Source: CAD feature listing. Evaluate the final solid. Frame: model axes, mm. Face numbers are marked on the shaded views. A direction names the side the tool comes from. Give positions to 0.01 mm unless a question says otherwise; leave off trailing zeros. Order: outer loops, then holes, each group sorted by start corner. A loop starts at its lowest first (then second) coordinate and runs counter-clockwise, first axis right, second up. Notation, with made-up numbers: (-3.5, 1) -> (40.5, 1) arc R21 cw to (40.5, 5) -> close; hole circle Ø10 at (14, 84.25). An arc over 180 degrees is marked (long way). Answer in a Markdown table with one row per item.
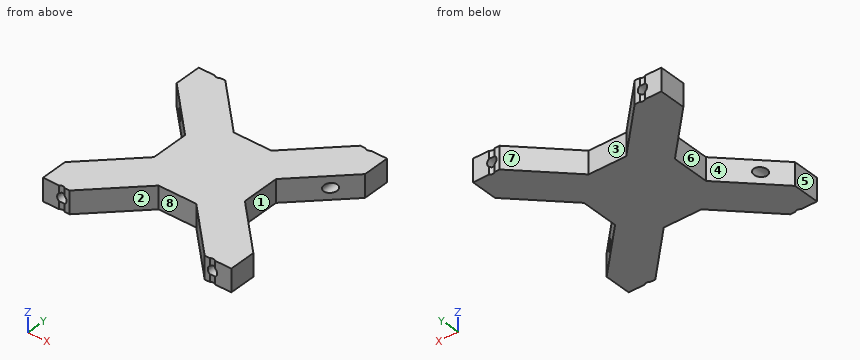
```python
from build123d import *

# Parameters (mm, degrees)
EXTRUDE_1_DEPTH        = 6
CUT_EXTRUDE_1_DEPTH    = 42.104177289
FILLET_1_R             = 2
FILLET_1_OF_MIRROR_3_R = 2
SKETCH_3_R             = 1.25
CUT_EXTRUDE_2_DEPTH    = 59.233427122
SKETCH_4_W             = 4.242640687
SKETCH_4_H             = 50
CUT_EXTRUDE_3_DEPTH    = 39.937540248


with BuildPart() as part:
    # ｽｹｯﾁ1 → ﾎﾞｽ - 押し出し1 (new body)
    with BuildSketch(Plane.XY):
        Polygon((-32.071067812, 25), (-12.071067812, 5), (-12.071067812, -5), (-32.071067812, -25), (-17.928932188, -25), (-5, -12.071067812), (5, -12.071067812), (17.928932188, -25), (32.071067812, -25), (12.071067812, -5), (12.071067812, 5), (32.071067812, 25), (17.928932188, 25), (5, 12.071067812), (-5, 12.071067812), (-17.928932188, 25), align=None)
    extrude(amount=EXTRUDE_1_DEPTH)

    # ｽｹｯﾁ2 → ｶｯﾄ - 押し出し1 (cut, through all)
    with BuildSketch(Plane.XY.offset(6)):
        with BuildLine():
            Line((-20.714142843, 25), (-19.285857157, 25))
            ThreePointArc((-19.285857157, 25), (-20, 24.7), (-20.714142843, 25))
        make_face()
        with BuildLine():
            Line((20.714142843, 25), (19.285857157, 25))
            ThreePointArc((19.285857157, 25), (20, 24.7), (20.714142843, 25))
        make_face()
    cut_extrude_1 = extrude(amount=-CUT_EXTRUDE_1_DEPTH, mode=Mode.SUBTRACT)

    # ﾌｨﾚｯﾄ1
    fillet_1_edges = [part.edges().sort_by_distance(p)[0] for p in [
        (32.071067812, 25, 3),
        (-32.071067812, 25, 3),
    ]]
    fillet(fillet_1_edges, radius=FILLET_1_R)

    # ﾐﾗｰ3: ｶｯﾄ - 押し出し1 across plane
    add(cut_extrude_1.mirror(Plane.ZX), mode=Mode.SUBTRACT)

    # ﾌｨﾚｯﾄ1 of ﾐﾗｰ3
    fillet_1_of_mirror_3_edges = [part.edges().sort_by_distance(p)[0] for p in [
        (32.071067812, -25, 3),
        (-32.071067812, -25, 3),
    ]]
    fillet(fillet_1_of_mirror_3_edges, radius=FILLET_1_OF_MIRROR_3_R)

    # ｽｹｯﾁ3 → ｶｯﾄ - 押し出し2 (cut, through all)
    with BuildSketch(Plane(origin=(0, 25, 0), x_dir=(1, 0, 0), z_dir=(0, 1, 0))):
        with Locations(Location((-20, -3, 0), (0, 0, 304.841925036))):
            Circle(SKETCH_3_R)
        with Locations(Location((20, -3, 0), (0, 0, 304.841925036))):
            Circle(SKETCH_3_R)
    extrude(amount=-CUT_EXTRUDE_2_DEPTH, mode=Mode.SUBTRACT)

    # ｽｹｯﾁ4 → ｶｯﾄ - 押し出し3 (cut, through all)
    with BuildSketch(Plane.XY.offset(6)):
        with Locations((-27.121320344, 0)):
            Rectangle(SKETCH_4_W, SKETCH_4_H)
        with Locations((27.121320344, 0)):
            Rectangle(SKETCH_4_W, SKETCH_4_H)
    extrude(amount=-CUT_EXTRUDE_3_DEPTH, mode=Mode.SUBTRACT)


solid = part.part
```
(1) Section query C-C (z = 5.25). Return the cut outline in (x, y).
A:
| item | result |
|---|---|
| outline | (-25, -25) -> (-20.71, -25) arc R1 cw to (-19.29, -25) -> (-17.93, -25) -> (-5, -12.07) -> (5, -12.07) -> (17.93, -25) -> (19.29, -25) arc R1 cw to (20.71, -25) -> (25, -25) -> (25, -17.93) -> (12.07, -5) -> (12.07, 5) -> (25, 17.93) -> (25, 25) -> (20.71, 25) arc R1 cw to (19.29, 25) -> (17.93, 25) -> (5, 12.07) -> (-5, 12.07) -> (-17.93, 25) -> (-19.29, 25) arc R1 cw to (-20.71, 25) -> (-25, 25) -> (-25, 17.93) -> (-12.07, 5) -> (-12.07, -5) -> (-25, -17.93) -> close |
(2) First-contact query: pin 1 Ø1.8 at (y, z) = (0.5, 2) entering from +X; pin 2 Ø3 at (x, z) = (-20, 3) entering from -Y; pin 3 Ø3 at (x, z) = (-0.5, 4.5) entering from -Y; pin 4 Ø1 at (y, z) = (-10.5, 2) entering from -X. Flat tips, straight axial feed; report the tip coordinate or a pass-through.
A:
| item | result |
|---|---|
| pin 1 | stops at x = 12.07 |
| pin 2 | stops at y = -25 |
| pin 3 | stops at y = -12.07 |
| pin 4 | stops at x = -18.07 |
(3) Section query D-D (y = -3.5). Return the cut outline in (x, z), plus the area to 3 significant figures.
A:
| item | result |
|---|---|
| outline | (-12.07, 0) -> (12.07, 0) -> (12.07, 6) -> (-12.07, 6) -> close |
| area | 145 mm^2 |
(4) Section query A-A (y = -19.5). Return the cut outline in (x, z), plus the area to 3 significant figures.
A:
| item | result |
|---|---|
| outline | (-25, 0) -> (-12.43, 0) -> (-12.43, 6) -> (-25, 6) -> close; (12.43, 0) -> (25, 0) -> (25, 6) -> (12.43, 6) -> close; hole circle Ø2.5 at (-20, 3); hole circle Ø2.5 at (20, 3) |
| area | 141 mm^2 |
(5) Access query for the marked faces 1, 2, 3 and 4. Directions: +Z, -Z, +X, -X, +Y, -Y. A direction counts if a zero-diameter tool reaches every point of the face in a straight line with its end or side. Return the directions, or none.
A:
| item | result |
|---|---|
| face 1 | +Z, -Z, +X |
| face 2 | +Z, -Z, -Y |
| face 3 | +Z, -Z, +Y |
| face 4 | +Z, -Z, -X |
(6) Ray query, probe 1 along Z at (x, y) = (20, -21.5); probe 2 along X at (y, z) = (-16.5, 3); probe 3 along X at (y, z) = (-16.25, 3). Return the intervals inside material, ascending.
A:
| item | result |
|---|---|
| probe 1 | z = 0 to 1.75, 4.25 to 6 |
| probe 2 | x = -23.57 to -21.25, -18.75 to -9.43, 9.43 to 18.75, 21.25 to 23.57 |
| probe 3 | x = -23.32 to -21.25, -18.75 to -9.18, 9.18 to 18.75, 21.25 to 23.32 |
(7) Section query B-B (x = 15.5). Return the cut outline in (y, z), plus the area to 3 significant figures.
A:
| item | result |
|---|---|
| outline | (-22.57, 0) -> (-8.43, 0) -> (-8.43, 6) -> (-22.57, 6) -> close; (8.43, 0) -> (22.57, 0) -> (22.57, 6) -> (8.43, 6) -> close |
| area | 170 mm^2 |
(8) Pull-direction query (Y, two-part tool) for the marked faces 5, 6, 7 and 8; classes: +Y half, -Y half, draft (parallel to the pull), parting line (faces both ways), or undercut.
A:
| item | result |
|---|---|
| face 5 | draft |
| face 6 | undercut |
| face 7 | +Y half |
| face 8 | -Y half |
